```python
from build123d import *

# Parameters (mm, degrees)
BOSS_EXTRUDE1_DEPTH = 15.24
CHAMFER1_SIZE       = 12.7
CHAMFER1_SIZE_2     = 120.832428569


with BuildPart() as part:
    # Sketch1 → Boss-Extrude1 (new body)
    with BuildSketch(Plane(origin=(0, 0, 0), x_dir=(1, 0, 0), z_dir=(0, 1, 0))):
        Polygon((0, 0), (177.8, 0), (177.8, 76.2), (127, 76.2), (127, 25.4), (0, 25.4), align=None)
    extrude(amount=BOSS_EXTRUDE1_DEPTH)

    # Chamfer1
    # the kernel refuses this chamfer: 120.832428569, 12.7 mm, written as the material it takes off along each edge
    with BuildSketch(Plane(origin=(-314.100660456, 15.24, 0), x_dir=(0, -0.9396808679591153, 0.34205243222582665), z_dir=(1, 0, 0))) as chamfer1_piece_1:
        Polygon((CHAMFER1_SIZE * 0.939680867959, CHAMFER1_SIZE * 0.342052432226), (-CHAMFER1_SIZE_2 * 0.342052432225, CHAMFER1_SIZE_2 * 0.939680867956), (0, 0), align=None)
    extrude(amount=806.001320912, mode=Mode.SUBTRACT)


solid = part.part
```
The model under review builds one solid part; all positions refer to its coordinate system, in mm. A direction names the side the tool comes from. Round coordinates to 2 decimals unless told otherwise and drop trailing zeros. Order: outer loops, then holes, each group sorted by start corner. A loop starts at its lowest first (then second) coordinate and runs counter-clockwise, first axis right, second up.
Item 1: For pin 1 (3 mm diameter, centred on y = 4.5, z = -38.5, fed in from -X); pin 2 (5 mm diameter, centred on x = 25.5, y = 9.5, fed in from -Z); pin 3 (1.6 mm diameter, centred on x = 40, y = 3, fed in from -Z); pin 4 (5 mm diameter, centred on x = 125.5, z = -67, fed in from +Y), all flat-tipped, find the tip position at first contact; note any pin that passes through.
Working result:
pin 1: stops at x = 127
pin 2: passes through
pin 3: stops at z = -25.4
pin 4: stops at y = 9.79
Item 2: Add section A-A, the plane z = -23. State the section outline as (x, y) points.
Working result:
outline: (0, 0) - (177.8, 0) - (177.8, 4.96) - (0, 4.96) - close
Item 3: To check wall thickness, follow probe 1 along X at (y, z) = (2.25, -45); probe 2 along Y at (x, z) = (131, -52.5); probe 3 along Z at (x, y) = (73.5, 1). State the ranges of each line that lie inside material, in increasing order.
Working result:
probe 1: x = 127 to 177.8
probe 2: y = 0 to 8.06
probe 3: z = -25.4 to 0
Item 4: Add section B-B, the plane x = 106.5. State the section outline as (y, z) points.
Working result:
outline: (0, -25.4) - (5.21, -25.4) - (2.54, 0) - (0, 0) - close
Item 5: Machinability: for faces 1 (the flat face through (64, 3, -25.4)), 2 (the flat face through (0, 2, -13)), which of the approach directions +Z, -Z, +X, -X, +Y, -Y give a long, thin tool a straight path to every point of the face, cutting with its end or side? Answer none if there is none.
Working result:
face 1: -Z, -X, +Y, -Y
face 2: +Z, -Z, -X, +Y, -Y
